Here's how the part is built. I have some questions about the finished solid (model axes, mm). A direction names the side the tool comes from. Coordinates: 2 decimals unless noted, no trailing zeros. Loops run counter-clockwise (first coordinate to the right, second up) from the corner with the lowest first, then second, coordinate; pieces in that order, holes last. Notation, with made-up numbers: M -4.5,27 L 27.5,27 A11 cw 27.5,31 Z; hole C 20,76.25 d8. An arc over 180 degrees is marked long. Use CSV: the item, a comma, the result in double quotes. Start each with the question number.
Q1. If we section it at B-B (z = 1.75): Please give me the cut outline in (x, y), and give its area (3 significant figures).
Q2. Which directions (+Z, -Z, +X, -X, +Y, -Y) give clear straight access to the entire face, cutting with the end or side of a thin tool? Please do faces 1 (the cylindrical face through (2.834, 33.667, -10.898)), 2 (the flat face through (6, 1.5, 0)).
Q3. For pin 1 Ø5 at (x, z) = (7.5, 11) entering from -Y; pin 2 Ø1.4 at (x, y) = (0.5, 9.5) entering from -Z; pin 3 Ø4 at (x, y) = (4, 27.5) entering from +Z; pin 4 Ø4 at (y, z) = (25.5, 5.5) entering from +X, each with a flat end and sliding along its axis, tell me the tip position at first contact or that it passes through.
Q4. If we section it at C-C (z = -8.5): Please give me the cut outline in (x, y), and give its area (3 significant figures).
Q5. If we section it at D-D (x = 4): Please give me the cut outline in (y, z), and give its area (3 significant figures).
Q6. Please list where these lines run through material, in increasing order: probe 1 along Z at (x, y) = (6, 34.05); probe 2 along Y at (x, z) = (3.5, 2); probe 3 along X at (y, z) = (10.5, 4.75). Write a range as [from, to].
Q7. If we section it at A-A (y = 17.25): Please give me the cut outline in (x, z).
Q8. If we mould it in two halves opening along Y, with no side actions, what happens to faces 3 (the flat face through (6, 0, 0)), 4 (the cylindrical face through (5.274, 0.761, -7.362)), 5 (the flat face through (6, 33, 0))? For each: +Y half, -Y half, draft (parallel to the pull), parting line (faces both ways), or undercut.
from build123d import *

# Parameters (mm, degrees)
BOSS_EXTRUDE1_DEPTH = 14
SKETCH2_R           = 1.35
CUT_EXTRUDE1_DEPTH  = 39.212694226
SKETCH4_R           = 1.742727666
CUT_EXTRUDE3_DEPTH  = 39.212694226
SKETCH3_R           = 3.5
CUT_EXTRUDE2_DEPTH  = 39.212694226
FILLET1_R           = 3
FILLET2_R           = 2
FILLET3_R           = 1.5


with BuildPart() as part:
    # Sketch1 → Boss-Extrude1 (new, symmetric)
    with BuildSketch(Plane.XY):
        Polygon((0, 0), (0, 34.5), (8.6, 34.5), (8.6, 33), (1.5, 33), (1.5, 1.5), (8.6, 1.5), (8.6, 0), align=None)
    extrude(amount=BOSS_EXTRUDE1_DEPTH, both=True)

    # Sketch2 → Cut-Extrude1 (cut, through all)
    with BuildSketch(Plane(origin=(0, 34.5, 0), x_dir=(1, 0, 0), z_dir=(0, 1, 0))):
        with Locations(Location((6, 8.5, 0), (0, 0, 180))):
            Circle(SKETCH2_R)
        with Locations(Location((6, -8.5, 0), (0, 0, 180))):
            Circle(SKETCH2_R)
    extrude(amount=-CUT_EXTRUDE1_DEPTH, mode=Mode.SUBTRACT)

    # Sketch4 → Cut-Extrude3 (cut, through all)
    with BuildSketch(Plane(origin=(0, 34.5, 0), x_dir=(1, 0, 0), z_dir=(0, 1, 0))):
        with BuildLine():
            Line((8.6, 14), (6, 14))
            ThreePointArc((6, 14), (7.838477631, 13.238477631), (8.6, 11.4))
            Line((8.6, 11.4), (8.6, 14))
        make_face()
        Polygon((0, 14.708926335), (0, 14), (1.742727666, 14), (6, 14), (8.6, 14), (8.6, 11.4), (10.428656455, 11.4), (10.428656455, 14.708926335), align=None)
        with BuildLine():
            ThreePointArc((3.485455332, 12.257272334), (3.47686088, 12.084409052), (3.451162292, 11.913250757))
            ThreePointArc((3.451162292, 11.913250757), (4.352949905, 13.411771852), (6, 14))
            Line((6, 14), (1.742727666, 14))
            ThreePointArc((1.742727666, 14), (2.975022216, 13.489566884), (3.485455332, 12.257272334))
        make_face()
        with Locations((1.742727666, 12.257272334)):
            Circle(SKETCH4_R)
        with BuildLine():
            Line((0, 14), (0, 12.257272334))
            ThreePointArc((0, 12.257272334), (0.510433116, 13.489566884), (1.742727666, 14))
            Line((1.742727666, 14), (0, 14))
        make_face()
        with BuildLine():
            Line((0, 10.514544668), (1.742727666, 10.514544668))
            ThreePointArc((1.742727666, 10.514544668), (0.510433116, 11.024977784), (0, 12.257272334))
            Line((0, 12.257272334), (0, 10.514544668))
        make_face()
    extrude(amount=-CUT_EXTRUDE3_DEPTH, mode=Mode.SUBTRACT)

    # Sketch3 → Cut-Extrude2 (cut, through all)
    with BuildSketch(Plane.ZY):
        with Locations((1.742727666, 17.25)):
            Circle(SKETCH3_R)
    extrude(amount=-CUT_EXTRUDE2_DEPTH, mode=Mode.SUBTRACT)

    # Fillet1
    fillet1_edges = [part.edges().sort_by_distance(p)[0] for p in [
        (0, 0, 1.742727666),
        (0, 34.5, 1.742727666),
    ]]
    fillet(fillet1_edges, radius=FILLET1_R)

    # Fillet2
    fillet2_edges = [part.edges().sort_by_distance(p)[0] for p in [
        (8.6, 33.75, 14),
        (8.6, 0.75, 14),
    ]]
    fillet(fillet2_edges, radius=FILLET2_R)

    # Fillet3
    fillet3_edges = [part.edges().sort_by_distance(p)[0] for p in [
        (1.5, 1.5, 1.742727666),
        (1.5, 33, 1.742727666),
    ]]
    fillet(fillet3_edges, radius=FILLET3_R)


solid = part.part
Results below:
1,outline,"M 0,3 A3 ccw 3,0 L 8.6,0 L 8.6,1.5 L 3,1.5 A1.5 cw 1.5,3 L 1.5,13.75 L 0,13.75 Z; M 0,20.75 L 1.5,20.75 L 1.5,31.5 A1.5 cw 3,33 L 8.6,33 L 8.6,34.5 L 3,34.5 A3 ccw 0,31.5 Z"
1,area,"59.7 mm^2"
2,face 1,"-Z, -X, +Y, -Y"
2,face 2,"+Z, -Z, +X"
3,pin 1,"y = 0"
3,pin 2,"z = -10.51"
3,pin 3,"through"
3,pin 4,"x = 1.5"
4,outline,"M 0,3 A3 ccw 3,0 L 4.65,0 L 4.65,1.5 L 3,1.5 A1.5 cw 1.5,3 L 1.5,31.5 A1.5 cw 3,33 L 4.65,33 L 4.65,34.5 L 3,34.5 A3 ccw 0,31.5 Z; M 7.35,0 L 8.6,0 L 8.6,1.5 L 7.35,1.5 Z; M 7.35,33 L 8.6,33 L 8.6,34.5 L 7.35,34.5 Z"
4,area,"62.1 mm^2"
5,outline,"M 0,-13.06 L 1.5,-13.06 L 1.5,14 L 0,14 Z; M 33,-13.06 L 34.5,-13.06 L 34.5,14 L 33,14 Z"
5,area,"81.2 mm^2"
6,probe 1,"[-14, -9.85], [-7.15, 7.15], [9.85, 14]"
6,probe 2,"[0, 1.5], [33, 34.5]"
6,probe 3,"[0, 1.5]"
7,outline,"M 0,-10.51 L 1.5,-10.51 L 1.5,-1.76 L 0,-1.76 Z; M 0,5.24 L 1.5,5.24 L 1.5,14 L 0,14 Z"
8,face 3,"-Y half"
8,face 4,"draft"
8,face 5,"undercut"
